```python
from build123d import *

# Parameters (mm, degrees)
F3_R     = 4.191
F3_R_2   = 2.921
F4_DEPTH = 50.8
F5_SIZE2 = 1.0208864232
F5_SIZE  = 3.81
F6_R     = 2.921
F7_DEPTH = 53.34


with BuildPart() as f1:
    # F0 (on Front) → F1 (revolve)
    with BuildSketch(Plane.XZ):
        Polygon((-3.81, 3.81), (0, 3.81), (3.81, 3.81), (16.51, 6.604), (41.91, 6.604), (41.91, 11.684), (16.51, 11.684), (3.81, 8.89), (0, 8.89), (-3.81, 8.89), (-16.51, 11.684), (-41.91, 11.684), (-41.91, 6.604), (-16.51, 6.604), align=None)
    revolve(axis=Axis((2.9206331819, 0, 0), (1, 0, 0)))

    # F3 (on offset) → F4 (join)
    with BuildSketch(Plane.XY.offset(3.81)):
        Circle(F3_R)
        Circle(F3_R_2, mode=Mode.SUBTRACT)
    extrude(amount=F4_DEPTH)

    # F5
    f5_edges = [f1.edges().sort_by_distance(p)[0] for p in [
        (-2.921, 0, 54.61),
    ]]
    f5_side = f1.faces().sort_by_distance((-2.921, 0, 31.503029))[0]
    chamfer(f5_edges, length=F5_SIZE, length2=F5_SIZE2, reference=f5_side)

    # F6 (on face) → F7 (cut)
    with BuildSketch(Plane.XY.offset(54.61)):
        Circle(F6_R)
    extrude(amount=-F7_DEPTH, mode=Mode.SUBTRACT)


solid = f1.part
```
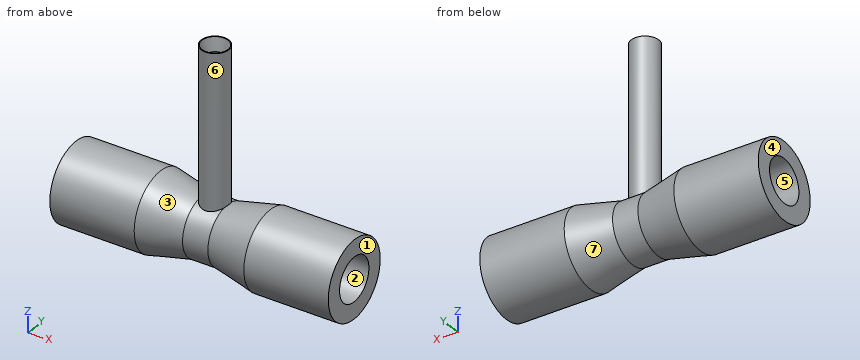
Part model, mm, in its own coordinate system. Face numbers are marked on the shaded views. A direction names the side the tool comes from. Round coordinates to 2 decimals unless told otherwise and drop trailing zeros. Order: outer loops, then holes, each group sorted by start corner. A loop starts at its lowest first (then second) coordinate and runs counter-clockwise, first axis right, second up. Notation, with made-up numbers: M 83,89 L 118,89 A9 cw 118,99 Z; hole C -17,38 d8. An arc over 180 degrees is marked long. Put each result on its own line as item: value. Start each with the question number.
1. Slice it at B-B on x = 0. List the corners of the cut face in (y, z).
2. Two-plate mould, pull along X, no slides. Class the marked faces 1, 2, 3 and 4: +X half, -X half, draft (parallel to the pull), parting line (faces both ways), or undercut.
3. Slice it at A-A on z = 0. List the corners of the cut face in (x, y), then the cut area to 3 significant figures.
4. Slice it at D-D on x = -9. List the corners of the cut face in (y, z), then the cut area to 3 significant figures.
5. Tool access for the marked faces 5, 6 and 7: list every direction of +Z, -Z, +X, -X, +Y, -Y with a clear straight run to the whole face (end or side of a thin tool).
6. Drop flat-ended pins along their axis: pin 1 (9.5 mm diameter, centred on x = 0, y = 0, fed in from +Z); pin 2 (3.5 mm diameter, centred on x = 0, y = 0, fed in from +Z); pin 3 (1 mm diameter, centred on x = 13, y = -5.5, fed in from -Z); pin 4 (12 mm diameter, centred on x = 6, y = -9, fed in from +Z). Give the stop position or say it passes through.
7. Drill centre lines: probe 1 along Y at (x, z) = (33.5, 0); probe 2 along Y at (x, z) = (0, 38); probe 3 along X at (y, z) = (0, 7.75). Where is each one in solid material? Low to high. Write a range as [from, to].
8. Slice it at C-C on x = -33.5. List the corners of the cut face in (y, z).
Findings:
1. outline: M -4.19,7.84 A8.89 ccw long 4.19,7.84 L 4.19,54.61 L 3.94,54.61 L 2.92,50.8 L 2.92,2.45 A3.81 cw long -2.92,2.45 L -2.92,50.8 L -3.94,54.61 L -4.19,54.61 Z
2. face 1: +X half
2. face 2: draft
2. face 3: undercut
2. face 4: -X half
3. outline: M -41.91,-11.68 L -16.51,-11.68 L -3.81,-8.89 L 3.81,-8.89 L 16.51,-11.68 L 41.91,-11.68 L 41.91,-6.6 L 16.51,-6.6 L 3.81,-3.81 L -3.81,-3.81 L -16.51,-6.6 L -41.91,-6.6 Z; M -41.91,6.6 L -16.51,6.6 L -3.81,3.81 L 3.81,3.81 L 16.51,6.6 L 41.91,6.6 L 41.91,11.68 L 16.51,11.68 L 3.81,8.89 L -3.81,8.89 L -16.51,11.68 L -41.91,11.68 Z
3. area: 852 mm2
4. outline: C 0,0 d20.06; hole C 0,0 d9.9
4. area: 239 mm2
5. face 5: -X
5. face 6: +Z
5. face 7: none
6. pin 1: z = 54.61
6. pin 2: z = -3.38
6. pin 3: z = -9.73
6. pin 4: z = 9.28
7. probe 1: [-11.68, -6.6], [6.6, 11.68]
7. probe 2: [-4.19, -2.92], [2.92, 4.19]
7. probe 3: [-41.91, -2.92], [2.92, 41.91]
8. outline: C 0,0 d23.37; hole C 0,0 d13.21
